Geometry: final body of the model. Coordinates: model frame, mm. A direction names the side the tool comes from. Coordinates: 2 decimals unless noted, no trailing zeros. Loops run counter-clockwise (first coordinate to the right, second up) from the corner with the lowest first, then second, coordinate; pieces in that order, holes last. Notation, with made-up numbers: (63, 62.5) - (100, 62.5) arc R25 cw to (100, 96.5) - close; hole circle Ø8 at (-0.5, -2.5). An arc over 180 degrees is marked (long way). Put each result on its own line as item: value. Start each with the question number.
1) Material intervals for line 1 along Y through (x, z) = (-18, 0); line 2 along Y through (x, z) = (37.5, 0.4); line 3 along X through (y, z) = (2.5, 2.5), sorted ascending. Write a range as from..to.
2) Reachability of faces 1 (the cylindrical face through (28.884, -0.867, 3.905)), 2 (the flat face through (34, 0, 1)), 3 (the flat face through (34, 0, -1)), 4 (the flat face through (0.5, 0, 0)), 5 (the flat face through (33, -3, 0)) from +Z, -Z, +X, -X, +Y, -Y: full face, straight path, thin tool, end or side. Return the list, or none.
3) Section A-A on y = 0. Output: boundary loops of the cut face in (x, z).
4) Contact query for flat-ended pins moving along their axis: pin 1 Ø2 at (y, z) = (-1.5, 1) entering from -X; pin 2 Ø1 at (x, z) = (33.5, 0.5) entering from -Y; pin 3 Ø2 at (x, z) = (27, -2) entering from -Y. Output: stop coordinate, or through.
5) Draft query along Y for faces 6 (the flat face through (34, 3, 0)), 7 (the cylindrical face through (-14, 0, 3)), 8 (the flat face through (-29.5, -1, -3)). Return one class per face: +Y half, -Y half, draft (parallel to the pull), parting line (faces both ways), or undercut.
6) Section C-C on x = -5.5. Output: boundary loops of the cut face in (y, z).
7) Section B-B on z = 0. Output: boundary loops of the cut face in (x, y), and give its area (3 significant figures).
8) Section D-D on x = 3. Output: boundary loops of the cut face in (y, z), and give its area (3 significant figures).
```python
from build123d import *

# Parameters (mm, degrees)
BOSS_EXTRUDE1_DEPTH          = 2
F_6_0_6_DIAMETER_HOLE1_D     = 6
F_6_0_6_DIAMETER_HOLE1_DEPTH = 30
F_5_0_5_DIAMETER_HOLE1_D     = 5
F_5_0_5_DIAMETER_HOLE1_DEPTH = 6.031754163


with BuildPart() as part:
    # Sketch1 → Revolve1 (revolve)
    with BuildSketch(Plane(origin=(0, 0, 0), x_dir=(-1, 0, 0), z_dir=(0, 0, -1))):
        with BuildLine():
            Line((-29.5, 4), (-29.5, 0))
            Line((-29.5, 0), (29.5, 0))
            Line((29.5, 0), (29.5, 4))
            Line((29.5, 4), (28.25, 4))
            ThreePointArc((28.25, 4), (27.515753003, 4.754613948), (26.5, 5.031754163))
            Line((26.5, 5.031754163), (-26.5, 5.031754163))
            ThreePointArc((-26.5, 5.031754163), (-27.515753003, 4.754613948), (-28.25, 4))
            Line((-28.25, 4), (-29.5, 4))
        make_face()
    revolve(axis=Axis((29.5, 0, 0), (-1, 0, 0)))

    # Sketch2 → Boss-Extrude1 (add)
    with BuildSketch(Plane.XY.offset(1)):
        with BuildLine():
            Line((37.5, 3), (29.5, 3))
            Line((29.5, 3), (29.5, -3))
            Line((29.5, -3), (37.5, -3))
            ThreePointArc((37.5, -3), (40.5, 0), (37.5, 3))
        make_face()
    extrude(amount=-BOSS_EXTRUDE1_DEPTH)

    # Ø6.0 (6) Diameter Hole1
    with Locations(Plane.ZY.offset(29.5)):
        with Locations((0, 0)):
            Hole(F_6_0_6_DIAMETER_HOLE1_D / 2, depth=F_6_0_6_DIAMETER_HOLE1_DEPTH)

    # Ø5.0 (5) Diameter Hole1
    with Locations(Plane(origin=(0, 0, -1), x_dir=(-1, 0, 0), z_dir=(0, 0, -1))):
        with Locations((-37.5, 0)):
            Hole(F_5_0_5_DIAMETER_HOLE1_D / 2, depth=F_5_0_5_DIAMETER_HOLE1_DEPTH)


solid = part.part
```
Answer block:
1. line 1: y = -5.03..-3, 3..5.03
1. line 2: y = -3..-2.5, 2.5..3
1. line 3: x = -29.5..29.5
2. face 1: +X
2. face 2: +Z, +X, +Y, -Y
2. face 3: -Z, +X, +Y, -Y
2. face 4: -X
2. face 5: +Z, -Z, +X, -Y
3. outline: (-29.5, -4) - (-28.25, -4) arc R2 ccw to (-26.5, -5.03) - (26.5, -5.03) arc R2 ccw to (28.25, -4) - (29.5, -4) - (29.5, -1) - (35, -1) - (35, 1) - (29.5, 1) - (29.5, 4) - (28.25, 4) arc R2 ccw to (26.5, 5.03) - (-26.5, 5.03) arc R2 ccw to (-28.25, 4) - (-29.5, 4) - (-29.5, 3) - (0.5, 3) - (0.5, -3) - (-29.5, -3) - close; (40, -1) - (40.5, -1) - (40.5, 1) - (40, 1) - close
4. pin 1: stops at x = 0.5
4. pin 2: stops at y = -3
4. pin 3: stops at y = -4.91
5. face 6: +Y half
5. face 7: undercut
5. face 8: draft
6. outline: circle Ø10.06 at (0, 0); hole circle Ø6 at (0, 0)
7. outline: (-29.5, -4) - (-28.25, -4) arc R2 ccw to (-26.5, -5.03) - (26.5, -5.03) arc R2 ccw to (28.25, -4) - (29.5, -4) - (29.5, -3) - (37.5, -3) arc R3 ccw to (37.5, 3) - (29.5, 3) - (29.5, 4) - (28.25, 4) arc R2 ccw to (26.5, 5.03) - (-26.5, 5.03) arc R2 ccw to (-28.25, 4) - (-29.5, 4) - (-29.5, 3) - (0.5, 3) - (0.5, -3) - (-29.5, -3) - close; hole circle Ø5 at (37.5, 0)
7. area: 449 mm²
8. outline: circle Ø10.06 at (0, 0)
8. area: 79.5 mm²
